from build123d import *

# Parameters (mm, degrees)
SKETCH2_W           = 355.6
SKETCH2_H           = 165.1
SKETCH2_R           = 31.75
SKETCH2_R_2         = 6.35
BOSS_EXTRUDE1_DEPTH = 3.175
CUT_EXTRUDE1_DEPTH  = 4.175


with BuildPart() as part:
    # Sketch2 → Boss-Extrude1 (new body)
    with BuildSketch(Plane.XY):
        with Locations((95.25, 0)):
            Rectangle(SKETCH2_W, SKETCH2_H)
        Circle(SKETCH2_R, mode=Mode.SUBTRACT)
        with Locations((-54.018973032, 17.551828308)):
            Circle(SKETCH2_R_2, mode=Mode.SUBTRACT)
        with Locations((0, 56.798909535)):
            Circle(SKETCH2_R_2, mode=Mode.SUBTRACT)
        with Locations((54.018973032, 17.551828308)):
            Circle(SKETCH2_R_2, mode=Mode.SUBTRACT)
        with Locations((33.385561371, -45.951283076)):
            Circle(SKETCH2_R_2, mode=Mode.SUBTRACT)
        with Locations((-33.385561371, -45.951283076)):
            Circle(SKETCH2_R_2, mode=Mode.SUBTRACT)
    extrude(amount=BOSS_EXTRUDE1_DEPTH)

    # Sketch3 → Cut-Extrude1 (cut, through all)
    with BuildSketch(Plane.XY.offset(3.175)):
        with BuildLine():
            Line((149.225, -9.525), (130.175, -9.525))
            ThreePointArc((130.175, -9.525), (127, -6.35), (130.175, -3.175))
            Line((130.175, -3.175), (149.225, -3.175))
            ThreePointArc((149.225, -3.175), (152.4, -6.35), (149.225, -9.525))
        make_face()
        with BuildLine():
            Line((250.825, -9.525), (231.775, -9.525))
            ThreePointArc((231.775, -9.525), (228.6, -6.35), (231.775, -3.175))
            Line((231.775, -3.175), (250.825, -3.175))
            ThreePointArc((250.825, -3.175), (254, -6.35), (250.825, -9.525))
        make_face()
        with BuildLine():
            Line((238.125, -60.325), (219.075, -60.325))
            ThreePointArc((219.075, -60.325), (215.9, -57.15), (219.075, -53.975))
            Line((219.075, -53.975), (238.125, -53.975))
            ThreePointArc((238.125, -53.975), (241.3, -57.15), (238.125, -60.325))
        make_face()
        with BuildLine():
            Line((142.875, -53.975), (161.925, -53.975))
            ThreePointArc((161.925, -53.975), (165.1, -57.15), (161.925, -60.325))
            Line((161.925, -60.325), (142.875, -60.325))
            ThreePointArc((142.875, -60.325), (139.7, -57.15), (142.875, -53.975))
        make_face()
    extrude(amount=-CUT_EXTRUDE1_DEPTH, mode=Mode.SUBTRACT)


solid = part.part
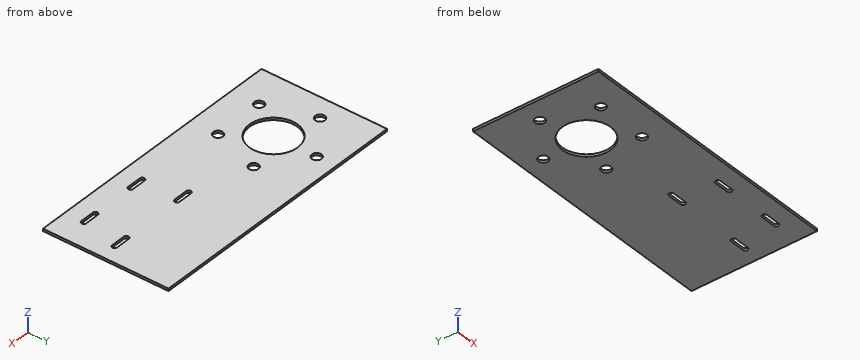
Could you check a few things on this model? Use its own coordinates, in mm. Give positions to 0.01 mm unless a question says otherwise; leave off trailing zeros. Order: outer loops, then holes, each group sorted by start corner. A loop starts at its lowest first (then second) coordinate and runs counter-clockwise, first axis right, second up. Notation, with made-up numbers: (50.25, 46.5) - (55.25, 46.5) arc R27 ccw to (55.25, 82.5) - close; hole circle Ø3 at (55.25, 0). An arc over 180 degrees is marked (long way). One line per question, with ' | ' between items. Start each with the question number.
Item 1: I'm going to push a flat-ended pin straight in: pin 1 Ø20.5 at (x, y) = (54.02, 17.55) entering from +Z (3 decimals). Where does the tip first touch, or does it pass through?
Item 2: I need wall thicknesses on probe 1 along Y at (x, z) = (146.5, 3) (3 decimals); probe 2 along Y at (x, z) = (0, 0.75); probe 3 along X at (y, z) = (-8, 0.4). Which ranges of each line are inside material? Lowest first, please. Write a range as [from, to].
Item 3: I want a section at D-D on z = 0.75. Give the number of separate pieces and of enclosed holes in the cut face, then the cut area to 3 significant figures.
Item 4: I want a section at C-C on y = 0. Write out the boundary of the cut face in (x, z) (3 decimals), then the cut area to 3 significant figures.
Item 5: I want a section at A-A on y = -57.15. Write out the boundary of the cut face in (x, z) (3 decimals).
Item 6: I want a section at B-B on x = 0. Write out the boundary of the cut face in (y, z) (3 decimals).
Verdict:
1) pin 1: z = 3.175
2) probe 1: [-82.55, -60.325], [-53.975, -9.525], [-3.175, 82.55] | probe 2: [-82.55, -31.75], [31.75, 50.45], [63.15, 82.55] | probe 3: [-82.55, -30.73], [30.73, 127.46], [151.94, 229.06], [253.54, 273.05]
3) separate pieces: 1 | enclosed holes: 10 | area: 54,300 mm^2
4) outline: (-82.55, 0) - (-31.75, 0) - (-31.75, 3.175) - (-82.55, 3.175) - close; (31.75, 0) - (273.05, 0) - (273.05, 3.175) - (31.75, 3.175) - close | area: 927 mm^2
5) outline: (-82.55, 0) - (139.7, 0) - (139.7, 3.175) - (-82.55, 3.175) - close; (165.1, 0) - (215.9, 0) - (215.9, 3.175) - (165.1, 3.175) - close; (241.3, 0) - (273.05, 0) - (273.05, 3.175) - (241.3, 3.175) - close
6) outline: (-82.55, 0) - (-31.75, 0) - (-31.75, 3.175) - (-82.55, 3.175) - close; (31.75, 0) - (50.449, 0) - (50.449, 3.175) - (31.75, 3.175) - close; (63.149, 0) - (82.55, 0) - (82.55, 3.175) - (63.149, 3.175) - close
